from build123d import *

# Parameters (mm, degrees)
F1_DEPTH = 254
F2_R     = 101.6


with BuildPart() as f1:
    # F0 (on Top) → F1 (new body)
    with BuildSketch(Plane.XY):
        Polygon((97.201592, 234.665401), (-97.201592, 234.665401), (-234.665401, 97.201592), (-234.665401, -97.201592), (-97.201592, -234.665401), (97.201592, -234.665401), (234.665401, -97.201592), (234.665401, 97.201592), align=None)
    extrude(amount=F1_DEPTH)

    # F2
    f2_edges = [f1.edges().sort_by_distance(p)[0] for p in [
        (0, 234.665401, 0),
        (-165.933497, 165.933497, 0),
        (-234.665401, 0, 0),
        (-165.933497, -165.933497, 0),
        (0, -234.665401, 0),
        (165.933497, -165.933497, 0),
        (234.665401, 0, 0),
        (165.933497, 165.933497, 0),
        (0, 234.665401, 254),
        (-165.933497, 165.933497, 254),
        (-234.665401, 0, 254),
        (-165.933497, -165.933497, 254),
        (0, -234.665401, 254),
        (165.933497, -165.933497, 254),
        (234.665401, 0, 254),
        (165.933497, 165.933497, 254),
    ]]
    fillet(f2_edges, radius=F2_R)


solid = f1.part
Source: CAD feature listing. Evaluate the final solid. Frame: model axes, mm. Coordinates: 2 decimals unless noted, no trailing zeros. Loops run counter-clockwise (first coordinate to the right, second up) from the corner with the lowest first, then second, coordinate; pieces in that order, holes last. Notation, with made-up numbers: (88, 24) -> (142, 24) arc R22 ccw to (142, 34) -> close; hole circle Ø1 at (-27, 8.25). An arc over 180 degrees is marked (long way). Answer in a Markdown table with one row per item. Add a question column.
Q1. Ray query, line 1 along Z through (x, y) = (114, -77.5); line 2 along X through (y, z) = (-55, 41); line 3 along Y through (x, z) = (145, 21.5). Return the intervals inside material, ascending.
Q2. Contact query for flat-ended pins moving along their axis: pin 1 Ø5 at (x, y) = (-147.5, -38) entering from +Z; pin 2 Ø5 at (x, y) = (-122.5, -156) entering from +Z; pin 3 Ø2 at (x, y) = (-132.5, -161) entering from -Z. Output: stop coordinate, or through.
Q3. Section B-B on x = 39. Return the cut outline in (y, z).
Q4. Section A-A on z = 144.5. Return the cut outline in (x, y).
Computed values:
| question | item | result |
|---|---|---|
| 1 | line 1 | z = 0.03 to 253.97 |
| 1 | line 2 | x = -214.61 to 214.61 |
| 1 | line 3 | y = -131.57 to 131.57 |
| 2 | pin 1 | stops at z = 253.3 |
| 2 | pin 2 | stops at z = 233.38 |
| 2 | pin 3 | stops at z = 31.42 |
| 3 | outline | (-234.67, 101.6) arc R101.6 ccw to (-133.07, 0) -> (133.07, 0) arc R101.6 ccw to (234.67, 101.6) -> (234.67, 152.4) arc R101.6 ccw to (133.07, 254) -> (-133.07, 254) arc R101.6 ccw to (-234.67, 152.4) -> close |
| 4 | outline | (-234.67, -97.2) -> (-97.2, -234.67) -> (97.2, -234.67) -> (234.67, -97.2) -> (234.67, 97.2) -> (97.2, 234.67) -> (-97.2, 234.67) -> (-234.67, 97.2) -> close |
